Build history of the part. All positions in model axes, mm. A direction names the side the tool comes from. Coordinates: 2 decimals unless noted, no trailing zeros. Loops run counter-clockwise (first coordinate to the right, second up) from the corner with the lowest first, then second, coordinate; pieces in that order, holes last. Notation, with made-up numbers: (78, 11) - (128, 11) arc R25 ccw to (128, 30) - close; hole circle Ø1 at (-21, 51.25). An arc over 180 degrees is marked (long way). One line per item, written item: value.
```python
from build123d import *

# Parameters (mm, degrees)
BOSS_EXTRUDE1_DEPTH        = 85
F_16_0_55_DIAMETER_HOLE1_D = 55
CUT_EXTRUDE1_DEPTH         = 85
FILLET1_RADIUS             = 42.5
FILLET1_LENGTH             = 20
F_16_0_16_DIAMETER_HOLE1_D = 16
F_16_0_16_DIAMETER_HOLE2_D = 16
SKETCH9_R                  = 3.5
CUT_EXTRUDE2_DEPTH         = 85
FILLET2_R                  = 15


with BuildPart() as part:
    # Sketch1 → Boss-Extrude1 (new body)
    with BuildSketch(Plane(origin=(0, 0, 0), x_dir=(0, 0, -1), z_dir=(1, 0, 0))):
        with BuildLine():
            ThreePointArc((-40.127920454, -14), (-42.5, 0), (-40.127920454, 14))
            Line((-40.127920454, 14), (-155, 14))
            Line((-155, 14), (-155, 10))
            Line((-155, 10), (-225, 10))
            Line((-225, 10), (-225, -10))
            Line((-225, -10), (-155, -10))
            Line((-155, -10), (-155, -14))
            Line((-155, -14), (-40.127920454, -14))
        make_face()
        with BuildLine():
            Line((36.806079661, 21.25), (0, 0))
            Line((0, 0), (0, -10))
            Line((0, -10), (0, -14))
            Line((0, -14), (-40.127920454, -14))
            ThreePointArc((-40.127920454, -14), (7.099766922, -41.902784032), (42.5, 0))
            ThreePointArc((42.5, 0), (41.051847617, 10.999809417), (36.806079661, 21.25))
        make_face()
        with BuildLine():
            Line((0, -10), (0, 0))
            Line((0, 0), (-8.082903769, 14))
            Line((-8.082903769, 14), (-40.127920454, 14))
            ThreePointArc((-40.127920454, 14), (-42.5, 0), (-40.127920454, -14))
            Line((-40.127920454, -14), (0, -14))
            Line((0, -14), (0, -10))
        make_face()
        with BuildLine():
            Line((-40.127920454, 14), (-8.082903769, 14))
            Line((-8.082903769, 14), (-12, 20.784609691))
            Line((-12, 20.784609691), (18.375771595, 38.322069598))
            ThreePointArc((18.375771595, 38.322069598), (-16.315016469, 39.243728641), (-40.127920454, 14))
        make_face()
        Polygon((-8.082903769, 14), (0, 0), (0, 10), (0, 14), align=None)
        with BuildLine():
            Line((0, 10), (0, 0))
            Line((0, 0), (36.806079661, 21.25))
            ThreePointArc((36.806079661, 21.25), (28.88118881, 31.178950157), (18.375771595, 38.322069598))
            Line((18.375771595, 38.322069598), (-12, 20.784609691))
            Line((-12, 20.784609691), (-8.082903769, 14))
            Line((-8.082903769, 14), (0, 14))
            Line((0, 14), (0, 10))
        make_face()
        with BuildLine():
            ThreePointArc((18.375771595, 38.322069598), (28.88118881, 31.178950157), (36.806079661, 21.25))
            Line((36.806079661, 21.25), (168.874953738, 97.5))
            Line((168.874953738, 97.5), (156.874953738, 118.284609691))
            Line((156.874953738, 118.284609691), (18.375771595, 38.322069598))
        make_face()
    extrude(amount=BOSS_EXTRUDE1_DEPTH)

    # Ø16.0 (55) Diameter Hole1 (through all)
    with Locations(Plane(origin=(85, 0, 0), x_dir=(0, 0, 1), z_dir=(1, 0, 0))):
        with Locations((0, 0)):
            Hole(F_16_0_55_DIAMETER_HOLE1_D / 2)

    # Sketch3 → Cut-Extrude1 (cut)
    with BuildSketch(Plane(origin=(0, 20.784609691, 12), x_dir=(1, 0, 0), z_dir=(0, 0.8660254037844386, 0.5000000000000002))):
        with BuildLine():
            Line((73, 127.58), (12, 127.58))
            Line((12, 127.58), (12, 127.579))
            ThreePointArc((12, 127.579), (14.343145751, 121.922145751), (20, 119.579))
            Line((20, 119.579), (65, 119.579))
            ThreePointArc((65, 119.579), (70.656854249, 121.922145751), (73, 127.579))
            Line((73, 127.579), (73, 127.58))
        make_face()
        with BuildLine():
            ThreePointArc((73, 106.369), (70.656854249, 100.712145751), (65, 98.369))
            Line((65, 98.369), (20, 98.369))
            ThreePointArc((20, 98.369), (14.343145751, 100.712145751), (12, 106.369))
            Line((12, 106.369), (12, 106.37))
            Line((12, 106.37), (73, 106.37))
            Line((73, 106.37), (73, 106.369))
        make_face()
        with BuildLine():
            ThreePointArc((73, 85.159), (70.656854249, 79.502145751), (65, 77.159))
            Line((65, 77.159), (20, 77.159))
            ThreePointArc((20, 77.159), (14.343145751, 79.502145751), (12, 85.159))
            Line((12, 85.159), (12, 85.16))
            Line((12, 85.16), (73, 85.16))
            Line((73, 85.16), (73, 85.159))
        make_face()
        with BuildLine():
            Line((73, 63.95), (12, 63.95))
            Line((12, 63.95), (12, 63.949))
            ThreePointArc((12, 63.949), (14.343145751, 58.292145751), (20, 55.949))
            Line((20, 55.949), (65, 55.949))
            ThreePointArc((65, 55.949), (70.656854249, 58.292145751), (73, 63.949))
            Line((73, 63.949), (73, 63.95))
        make_face()
        with BuildLine():
            Line((12, 170), (73, 170))
            Line((73, 170), (73, 169.999))
            ThreePointArc((73, 169.999), (70.656854249, 164.342145751), (65, 161.999))
            Line((65, 161.999), (20, 161.999))
            ThreePointArc((20, 161.999), (14.343145751, 164.342145751), (12, 169.999))
            Line((12, 169.999), (12, 170))
        make_face()
        with BuildLine():
            Line((73, 148.79), (12, 148.79))
            Line((12, 148.79), (12, 148.789))
            ThreePointArc((12, 148.789), (14.343145751, 143.132145751), (20, 140.789))
            Line((20, 140.789), (65, 140.789))
            ThreePointArc((65, 140.789), (70.656854249, 143.132145751), (73, 148.789))
            Line((73, 148.789), (73, 148.79))
        make_face()
    extrude(amount=-CUT_EXTRUDE1_DEPTH, mode=Mode.SUBTRACT)

    # Fillet1: full round fillet: the end face becomes a half cylinder, R = half its width
    fillet1_face = Plane((42.5, 0, 225), x_dir=(0, -1, 0), z_dir=(0, 0, 1))  # on the end face: x along it, z out of the body
    fillet1_slab = fillet1_face.offset(-FILLET1_RADIUS / 2) * Box(FILLET1_LENGTH, 2 * FILLET1_RADIUS, FILLET1_RADIUS, mode=Mode.PRIVATE)  # the body's end, R deep
    fillet1_round = Plane((42.5, 0, 182.5), x_dir=(0, 0, 1), z_dir=(0, -1, 0)) * Cylinder(FILLET1_RADIUS, FILLET1_LENGTH, mode=Mode.PRIVATE)  # its axis R under the face
    add(fillet1_slab - fillet1_round, mode=Mode.SUBTRACT)

    # Ø16.0 (16) Diameter Hole1 (through all)
    with Locations(Plane(origin=(42.5, -10, 182.5), x_dir=(0, 0, -1), z_dir=(0, -1, 0))):
        with Locations((0, 0)):
            Hole(F_16_0_16_DIAMETER_HOLE1_D / 2)

    # Ø16.0 (16) Diameter Hole2 (through all)
    with Locations(Plane(origin=(42.5, 14, 97.563960227), x_dir=(0, 0, 1), z_dir=(0, 1, 0))):
        with Locations((0, 0)):
            Hole(F_16_0_16_DIAMETER_HOLE2_D / 2)

    # Sketch9 → Cut-Extrude2 (cut)
    with BuildSketch(Plane(origin=(0, 14, 0), x_dir=(1, 0, 0), z_dir=(0, 1, 0))):
        with Locations(Location((42.5, -72.563960227, 0), (0, 0, 270))):
            Circle(SKETCH9_R)
        with Locations(Location((64.150635095, -85.063960227, 0), (0, 0, 270))):
            Circle(SKETCH9_R)
        with Locations(Location((64.150635095, -110.063960227, 0), (0, 0, 270))):
            Circle(SKETCH9_R)
        with Locations(Location((42.5, -122.563960227, 0), (0, 0, 270))):
            Circle(SKETCH9_R)
        with Locations(Location((20.849364905, -110.063960227, 0), (0, 0, 270))):
            Circle(SKETCH9_R)
        with Locations(Location((20.849364905, -85.063960227, 0), (0, 0, 270))):
            Circle(SKETCH9_R)
    extrude(amount=-CUT_EXTRUDE2_DEPTH, mode=Mode.SUBTRACT)

    # Fillet2
    fillet2_edges = [part.edges().sort_by_distance(p)[0] for p in [
        (85, 107.892304845, -162.874953738),
        (0, 107.892304845, -162.874953738),
    ]]
    fillet(fillet2_edges, radius=FILLET2_R)


solid = part.part
```
Item 1: Pull direction X, two halves, no side cores. Call faces 4 (the face through (51, 14, 97)), 5 (the face through (42.073, 53.118, -67.667)), 6 (the face through (85, 29, 14)): released by +X, released by -X, zero draft, split by the parting line, or undercut.
Check result:
face 4: zero draft
face 5: undercut
face 6: released by +X
Item 2: Tool access for faces 1 (the face through (42.07, 95.54, -141.14)), 2 (the face through (51, -10, 183)), 3 (the face through (51, 10, 190)): list every direction of +Z, -Z, +X, -X, +Y, -Y with a clear straight run to the whole face (end or side of a thin tool).
Check result:
face 1: none
face 2: +Z, +X, -X, -Y
face 3: +Z, +X, -X, +Y
Item 3: Cut at A-A, the plane z = 0. Write the cut outline in (x, y), then the cut area to 3 significant figures.
Check result:
outline: (0, -42.5) - (85, -42.5) - (85, -27.5) - (0, -27.5) - close; (0, 27.5) - (85, 27.5) - (85, 42.5) - (0, 42.5) - close
area: 2,550 mm^2
Item 4: Drop flat-ended pins along their axis: P1, Ø5, axis at x = 74, y = 16, coming from the +Z side; P2, Ø6, axis at x = 55, z = 136.5, coming from the +Y side; P3, Ø18.5, axis at x = 42.5, z = 97.56, coming from the -Y side; P4, Ø4, axis at x = 64.15, z = 85.06, coming from the -Y side. Give the stop position or say it passes through.
Check result:
P1: stops at z = 155
P2: stops at y = 14
P3: stops at y = -14
P4: passes through
Item 5: Cut at B-B, the plane x = 42.5. Give the number of separate pieces and of enclosed holes in the cut face, then the cut area to 3 significant figures.
Check result:
separate pieces: 11
enclosed holes: 1
area: 9,280 mm^2
Item 6: Cut at C-C, the plane z = 101.5. Write the cut outline in (x, y), then the cut area to 3 significant figures.
Check result:
outline: (0, -14) - (35.54, -14) - (35.54, 14) - (0, 14) - close; (49.46, -14) - (85, -14) - (85, 14) - (49.46, 14) - close
area: 1,990 mm^2
Item 7: Probe probe 1 along Z at (x, y) = (52, 64); probe 2 along Z at (x, y) = (36, -1.5); probe 3 along Y at (x, z) = (45.5, 0). List the from-to ranges inside material, lowest first. Write a range as from..to.
Check result:
probe 1: z = -110.85..-110.37, -101.13..-85.88, -76.64..-62.85
probe 2: z = -42.47..-27.46, 27.46..92.9, 102.23..177.84, 187.16..224.5
probe 3: y = -42.5..-27.5, 27.5..42.5
